```python
from build123d import *

# Parameters (mm, degrees)
F0_R     = 1.6
F0_R_2   = 6
F0_R_3   = 4
F0_R_4   = 1.75
F0_R_5   = 10
F1_DEPTH = 30


# Not quite as in the source:
# - ends of sketch curves that miss each other by under 0.0002 mm in the source are joined


with BuildPart() as f1:
    # F0 (on Right) → F1 (new body)
    with BuildSketch(Plane.YZ):
        with BuildLine():
            Line((191, -122.083788), (191, -49.632945))
            ThreePointArc((191, -49.632945), (188.7918883648, -32.5816457168), (182.3132286148, -16.6552672181))
            Line((182.3132286148, -16.6552672181), (112.877133, 106))
            Line((112.877133, 106), (105.625999, 118.808753))
            ThreePointArc((105.625999, 118.808753), (89.4861101441, 131.177974009), (69.378816691, 128.1464075024))
            Line((69.378816691, 128.1464075024), (-174.970501, -22.141031))
            ThreePointArc((-174.970501, -22.141031), (-186.7206628889, -34.3919513631), (-191, -50.818717))
            Line((-191, -50.818717), (-191, -122.083788))
            ThreePointArc((-191, -122.083788), (-188.0956097489, -129.0956087489), (-181.083789, -132))
            Line((-181.083789, -132), (83, -132))
            Line((83, -132), (181.083788, -132))
            ThreePointArc((181.083788, -132), (188.0956087489, -129.0956087489), (191, -122.083788))
        make_face()
        with Locations((-171, -114.5)):
            Circle(F0_R, mode=Mode.SUBTRACT)
        with Locations((-171, -99.5)):
            Circle(F0_R, mode=Mode.SUBTRACT)
        with Locations((-151, -114.5)):
            Circle(F0_R, mode=Mode.SUBTRACT)
        with Locations((-151, -99.5)):
            Circle(F0_R, mode=Mode.SUBTRACT)
        with Locations((-171, -64.5)):
            Circle(F0_R, mode=Mode.SUBTRACT)
        with Locations((-151, -64.5)):
            Circle(F0_R, mode=Mode.SUBTRACT)
        with Locations((-171, -49.5)):
            Circle(F0_R, mode=Mode.SUBTRACT)
        with Locations((-151, -49.5)):
            Circle(F0_R, mode=Mode.SUBTRACT)
        with Locations((151, -114.5)):
            Circle(F0_R, mode=Mode.SUBTRACT)
        with Locations((151, -99.5)):
            Circle(F0_R, mode=Mode.SUBTRACT)
        with Locations((171, -114.5)):
            Circle(F0_R, mode=Mode.SUBTRACT)
        with Locations((171, -99.5)):
            Circle(F0_R, mode=Mode.SUBTRACT)
        with Locations((72.000954, -12.999046)):
            Circle(F0_R, mode=Mode.SUBTRACT)
        with Locations((83, -2)):
            Circle(F0_R_2, mode=Mode.SUBTRACT)
        with Locations((151, -64.5)):
            Circle(F0_R, mode=Mode.SUBTRACT)
        with Locations((171, -64.5)):
            Circle(F0_R, mode=Mode.SUBTRACT)
        with Locations((151, -49.5)):
            Circle(F0_R, mode=Mode.SUBTRACT)
        with Locations((171, -49.5)):
            Circle(F0_R, mode=Mode.SUBTRACT)
        with Locations((162.986451, -5.858929)):
            Circle(F0_R_3, mode=Mode.SUBTRACT)
        with Locations((93.999046, 8.999046)):
            Circle(F0_R, mode=Mode.SUBTRACT)
        with Locations((67.443651, 21.443651)):
            Circle(F0_R_4, mode=Mode.SUBTRACT)
        with Locations((83, 21.445)):
            Circle(F0_R, mode=Mode.SUBTRACT)
        with Locations((67.445, 37)):
            Circle(F0_R, mode=Mode.SUBTRACT)
        with Locations((83, 37)):
            Circle(F0_R_5, mode=Mode.SUBTRACT)
        with Locations((67.443651, 52.556349)):
            Circle(F0_R_4, mode=Mode.SUBTRACT)
        with Locations((83, 52.555)):
            Circle(F0_R, mode=Mode.SUBTRACT)
        with Locations((72.000954, 65.000954)):
            Circle(F0_R, mode=Mode.SUBTRACT)
        with Locations((98.556349, 21.443651)):
            Circle(F0_R_4, mode=Mode.SUBTRACT)
        with Locations((98.555, 37)):
            Circle(F0_R, mode=Mode.SUBTRACT)
        with Locations((98.556349, 52.556349)):
            Circle(F0_R_4, mode=Mode.SUBTRACT)
        with Locations((83, 76)):
            Circle(F0_R_2, mode=Mode.SUBTRACT)
        with Locations((93.999046, 86.999046)):
            Circle(F0_R, mode=Mode.SUBTRACT)
        with Locations((113.720248, 81.167269)):
            Circle(F0_R_3, mode=Mode.SUBTRACT)
    extrude(amount=F1_DEPTH)


solid = f1.part
```
Read the model definition and answer for the solid it produces. Units are mm, in the model's axes. Coordinates: 2 decimals unless noted, no trailing zeros. Loops run counter-clockwise (first coordinate to the right, second up) from the corner with the lowest first, then second, coordinate; pieces in that order, holes last. Notation, with made-up numbers: (56.5, -26.5) -> (80.5, -26.5) arc R22 cw to (80.5, -15.5) -> close; hole circle Ø5 at (5, 84.5). An arc over 180 degrees is marked (long way). Return JSON: item names as keys, results as strings.
Item 1: Flat-ended cylindrical pins translate along their axes: P1, Ø3.5, axis at y = -151, z = -49.5, coming from the +X side; P2, Ø1.5, axis at x = 15, y = 33.5, coming from the +Z side; P3, Ø6, axis at x = 7.5, y = -35, coming from the +Z side; P4, Ø1, axis at x = 8.5, z = 100.5, coming from the -Y side. Find the tip coordinate at first contact, or state that the pin passes through.
Answers:
{"P1": "stops at x = 30", "P2": "stops at z = 106.54", "P3": "stops at z = 65.79", "P4": "stops at y = 23.62"}
Item 2: Find the intervals of material crossed by probe 1 along Y at (x, z) = (8.75, -114.5); probe 2 along Y at (x, z) = (17, -4); probe 3 along Z at (x, y) = (22.25, 171), in increasing order.
Answers:
{"probe 1": "y = -191 to -172.6, -169.4 to -152.6, -149.4 to 149.4, 152.6 to 169.4, 172.6 to 191", "probe 2": "y = -145.48 to 77.34, 88.66 to 159.44, 166.53 to 175.15", "probe 3": "z = -132 to -116.1, -112.9 to -101.1, -97.9 to -66.1, -62.9 to -51.1, -47.9 to 3.33"}
Item 3: Find section B-B (y = 29). Determine the outline of the cut face in (x, z), plus the area to 3 significant figures.
Answers:
{"outline": "(0, -132) -> (30, -132) -> (30, 103.31) -> (0, 103.31) -> close", "area": "7,060 mm2"}
Item 4: Find section A-A (y = -111). Determine the outline of the cut face in (x, z).
Answers:
{"outline": "(0, -132) -> (30, -132) -> (30, 17.2) -> (0, 17.2) -> close"}
Item 5: For a pull along Y with two mould halves and no side action, classify faces 1 (the cylindrical face through (14.79, 78.58, 80.06)), 2 (the flat face through (15, -191, -86)), 3 (the cylindrical face through (14.79, 188.853, -32.815)) as +Y half, -Y half, draft (parallel to the pull), parting line (faces both ways), or undercut.
Answers:
{"face 1": "undercut", "face 2": "-Y half", "face 3": "+Y half"}
